Can you work these out from the model? Positions are in its coordinate system, mm. A direction names the side the tool comes from. Give positions to 0.01 mm unless a question says otherwise; leave off trailing zeros. Write each loop counter-clockwise with the first axis right and the second up, starting at its lowest first coordinate (ties: lowest second). Pieces come first, ordered by that corner, then holes.
1. On a 3-axis mill with a long thin cutter (end or side, diameter ignored), from which of +Z, -Z, +X, -X, +Y, -Y can I reach the whole of each face in a straight line? I mean faces 4 (the flat face through (0, 3, -2.424)), 5 (the flat face through (0, 3, -3.424)). Say none if no direction works.
2. Suppose I cut it at B-B (z = 0.7). Please give me the cut outline in (x, y).
3. Suppose I cut it at D-D (x = -0.15). Please give me the cut outline in (y, z).
4. Suppose I cut it at C-C (x = 0.4). Please give me the cut outline in (y, z).
5. If I drill on probe 1 along X at (y, z) = (4.75, -3.15); probe 2 along Z at (x, y) = (-0.6, 2.25); probe 3 along X at (y, z) = (6, -2.95), over which ranges is the centre line in solid material (lowest first)?
6. Thinking about a two-plate mould opening in Z: for faces 1 (the flat face through (0, 7, -3)), 2 (the flat face through (-0.3, 0.5, 2.576)), 3 (the cylindrical face through (-1.77, 0.49, -0.12)), which applies, pulls with the +Z half, pulls with the -Z half, needs draft (parallel to the pull), parting line crosses it, or undercut?
7. I'm going to push a flat-ended pin straight in: pin 1 (1 mm diameter, centred on x = -2, y = 5.5, fed in from +Z). Where does the tip first touch, or does it pass through?
8. Suppose I cut it at A-A (y = 4.75). Please give me the cut outline in (x, z).
Autodesk Inventor part; units mm, degrees
ref_plane "YZ Plane" through (0, 0, 0) normal (1, 0, 0) x (0, 1, 0)
ref_plane "XZ Plane" through (0, 0, 0) normal (0, 1, 0) x (-1, 0, 0)
ref_plane "XY Plane" through (0, 0, 0) normal (0, 0, 1) x (1, 0, 0)
sketch "Sketch1" plane through (0, 0, 0) normal (0, 1, 0) x (-1, 0, 0)
  line L0 (-1.9318, 2.5757) -> (2.5682, 2.5757)
  line L1 (2.5682, 2.5757) -> (2.5682, -3.4243)
  line L2 (2.5682, -3.4243) -> (-1.9318, -3.4243)
  line L3 (-1.9318, -3.4243) -> (-1.9318, 2.5757)
  line L4 (-1.9318, 2.5757) -> (2.5682, -3.4243) construction
  circle A0 centre (0.3372, 0.3257) radius 1.5
  point P0 (0, 0)
  dimension "d0" = 4.5
  dimension "d1" = 6
  dimension "d3" = 2.25
extrude "Extrusion1" add sketch "Sketch1" along normal blind 1
sketch "Sketch2" plane through (0, 1, 0) normal (0, 1, 0) x (1, 0, 0)
  circle A0 centre (-0.3372, -0.3257) radius 1.5
  line L0 (-2.5682, -2.5757) -> (1.9318, -2.5757)
  line L1 (1.9318, -2.5757) -> (1.9318, 3.4243)
  line L2 (1.9318, 3.4243) -> (-2.5682, 3.4243)
  line L3 (-2.5682, 3.4243) -> (-2.5682, -2.5757)
  line L4 (-2.5682, 3.4243) -> (-2.5682, -2.5757)
  line L5 (-2.5682, 3.4243) -> (-2.5682, 2.4243)
  line L6 (-2.5682, 2.4243) -> (1.9318, 2.4243)
  line L7 (1.9318, 2.4243) -> (1.9318, 3.4243)
  line L8 (1.9318, 3.4243) -> (-2.5682, 3.4243)
  dimension "d6" = 1
extrude "Extrusion2" add sketch "Sketch2" along normal blind 6 contours L3 L2 L1 L6
fillet "Fillet1" radius 1.5 1 edges at (-0.3182, 0, -3.4243)
sketch "Sketch3" plane through (1.9318, 7, -3.4243) normal (0, 0, -1) x (-1, 0, 0)
  line L0 (4.5, -5.5) -> (0, -5.5)
  line L1 (4.5, -5.5) -> (4.5, 0)
  line L2 (0, 0) -> (4.5, 0)
  line L3 (0, -5.5) -> (0, 0)
  line L4 (2.25, 0) -> (2.25, -2.25)
  circle A0 centre (2.25, -2.25) radius 1.5
  point P0 (1.9318, -7)
  dimension "d10" = 2.25
  dimension "d11" = 3
extrude "Extrusion3" cut sketch "Sketch3" against normal blind 6 contours A0
fillet "Fillet2" radius 0.5 1 edges at (-0.3182, 1, -2.4243)
properties part number "Pixy angle bracket"
Checks:
1. face 4: +Z, +X, -X, +Y
1. face 5: -Z, +X, -X, +Y, -Y
2. outline: (-2.57, 0) - (-1.79, 0) - (-1.79, 1) - (-2.57, 1) - close; (1.12, 0) - (1.93, 0) - (1.93, 1) - (1.12, 1) - close
3. outline: (0, -1.92) arc R1.5 ccw to (1.5, -3.42) - (3.26, -3.42) - (3.26, -2.42) - (1.5, -2.42) arc R0.5 cw to (1, -1.92) - (1, -1.16) - (0, -1.16) - close; (0, 1.81) - (1, 1.81) - (1, 2.58) - (0, 2.58) - close; (6.24, -3.42) - (7, -3.42) - (7, -2.42) - (6.24, -2.42) - close
4. outline: (0, -1.92) arc R1.5 ccw to (1.5, -3.42) - (3.43, -3.42) - (3.43, -2.42) - (1.5, -2.42) arc R0.5 cw to (1, -1.92) - (1, -0.98) - (0, -0.98) - close; (0, 1.63) - (1, 1.63) - (1, 2.58) - (0, 2.58) - close; (6.07, -3.42) - (7, -3.42) - (7, -2.42) - (6.07, -2.42) - close
5. probe 1: x = -2.57 to -1.82, 1.18 to 1.93
5. probe 2: z = -3.42 to -2.42
5. probe 3: x = -2.57 to -1.15, 0.51 to 1.93
6. face 1: needs draft
6. face 2: pulls with the +Z half
6. face 3: undercut
7. pin 1: stops at z = -2.42
8. outline: (-2.57, -3.42) - (-1.82, -3.42) - (-1.82, -2.42) - (-2.57, -2.42) - close; (1.18, -3.42) - (1.93, -3.42) - (1.93, -2.42) - (1.18, -2.42) - close
